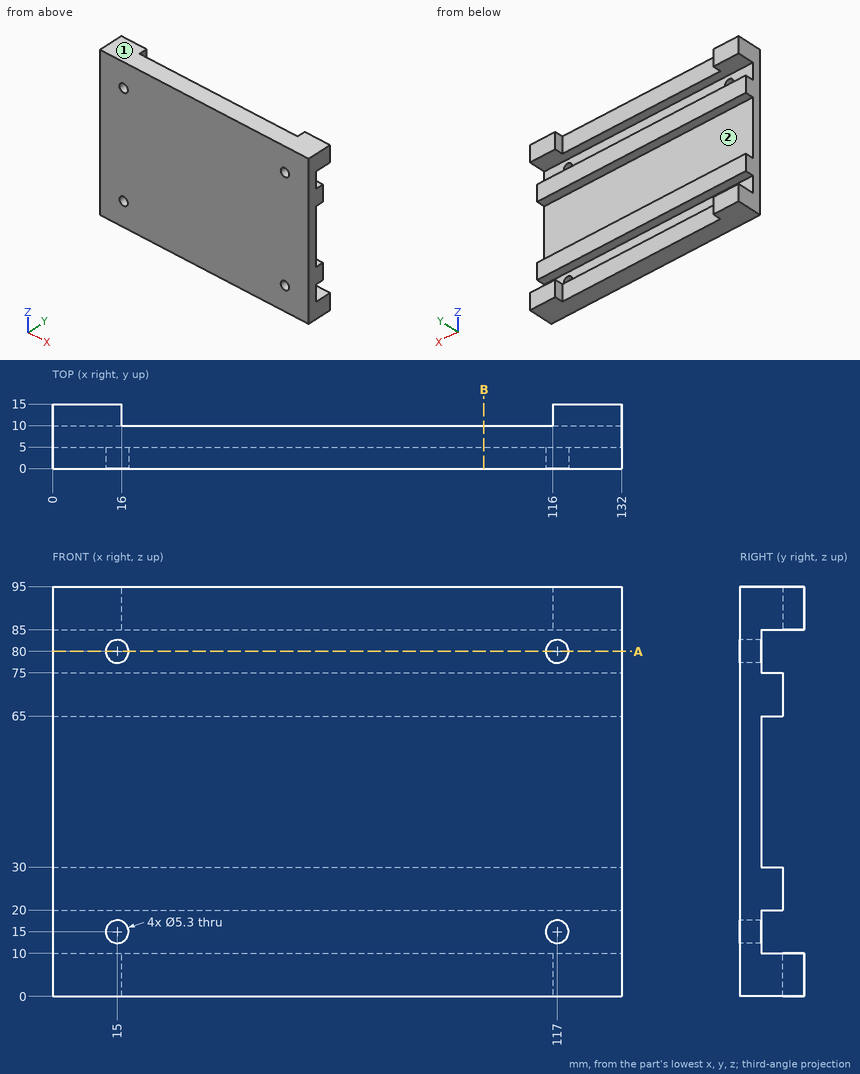
Can you work these out from the drawing? Everything is in mm from the part's minimum corner. A direction names the side the tool comes from. Round coordinates to 2 decimals unless told otherwise and drop trailing zeros. Loops run counter-clockwise (first coordinate to the right, second up) from the corner with the lowest first, then second, coordinate; pieces in that order, holes last. Notation, with made-up numbers: (-30.75, -36.75) - (25.25, -36.75) arc R12 cw to (25.25, -27.75) - close; hole circle Ø3 at (57, 74.25). An arc over 180 degrees is marked (long way). One line per question, with ' | ' between items. Start each with the question number.
Q1. I want a section at B-B (x = 100). Write out the boundary of the cut face in (y, z), then the cut area to 3 significant figures.
Q2. For the marked faces 1 and 2, which set-ups out of +Z, -Z, +X, -X, +Y, -Y let a thin tool reach every point of the face, with its end or its side?
Q3. Will these pins go through, and if not, where does the flat tip stop? pin 1 (1 mm diameter, centred on x = 45, y = 10, fed in from -Z); pin 2 (3 mm diameter, centred on x = 52, z = 13.5, fed in from +Y); pin 3 (8 mm diameter, centred on x = 76, z = 68, fed in from +Y); pin 4 (4 mm diameter, centred on x = 34, y = 12.5, fed in from -Z).
Q4. Please list where these lines run through material, in increasing order: line 1 (Z direction, x = 117, y = 2.6); line 2 (X direction, y = 3.5, z = 80); line 3 (Z direction, x = 11, y = 8.75). Write a range as [from, to].
Q5. I want a section at A-A (z = 80). Write out the boundary of the cut face in (x, y).
Response values:
1) outline: (0, 0) - (10, 0) - (10, 10) - (5, 10) - (5, 20) - (10, 20) - (10, 30) - (5, 30) - (5, 65) - (10, 65) - (10, 75) - (5, 75) - (5, 85) - (10, 85) - (10, 95) - (0, 95) - close | area: 675 mm²
2) face 1: +Z, +X, -X, +Y, -Y | face 2: +X, -X, +Y
3) pin 1: stops at z = 0 | pin 2: stops at y = 5 | pin 3: stops at y = 10 | pin 4: passes through
4) line 1: z = [0, 12.35], [17.65, 77.35], [82.65, 95] | line 2: x = [0, 12.35], [17.65, 114.35], [119.65, 132] | line 3: z = [0, 10], [20, 30], [65, 75], [85, 95]
5) outline: (0, 0) - (12.35, 0) - (12.35, 5) - (0, 5) - close; (17.65, 0) - (114.35, 0) - (114.35, 5) - (17.65, 5) - close; (119.65, 0) - (132, 0) - (132, 5) - (119.65, 5) - close
